Check sheet for the modelled part. Datum: model origin and axes. Units: mm. A direction names the side the tool comes from. Give positions to 0.01 mm unless a question says otherwise; leave off trailing zeros. Order: outer loops, then holes, each group sorted by start corner. A loop starts at its lowest first (then second) coordinate and runs counter-clockwise, first axis right, second up. Notation, with made-up numbers: M -8.75,64.25 L 29.25,64.25 A12 cw 29.25,71.25 Z; hole C 54,79.25 d3. An arc over 180 degrees is marked long. Answer in a Markdown table with one row per item. Add a question column.
from build123d import *

# Parameters (mm, degrees)
ESQUISSE1_W               = 99.5
ESQUISSE1_H               = 12.5
ESQUISSE2_W               = 4.8
ESQUISSE2_H               = 5
ENL_V_MAT_EXTRU_1_DEPTH   = 13.5
SYM_TRIE2_COPY_1_SKETCH_W = 4.8
SYM_TRIE2_COPY_1_SKETCH_H = 5
SYM_TRIE2_COPY_1_DEPTH    = 13.5


with BuildPart() as part:
    # Esquisse1 → Révolution1 (revolve)
    with BuildSketch(Plane.XY, mode=Mode.PRIVATE) as r_volution1_sk:
        with Locations((0, 6.25)):
            Rectangle(ESQUISSE1_W, ESQUISSE1_H)
    revolve(r_volution1_sk.sketch.rotate(Axis((-69.457729469, 0, 0), (1, 0, 0)), 90), axis=Axis((-69.457729469, 0, 0), (1, 0, 0)))  # turned: the seam where the file's is

    # Esquisse2 → Enlèv. mat.-Extru.1 (cut, symmetric)
    with BuildSketch(Plane.XY):
        with Locations((-47.35, 10)):
            Rectangle(ESQUISSE2_W, ESQUISSE2_H)
    enl_v_mat_extru_1 = extrude(amount=ENL_V_MAT_EXTRU_1_DEPTH, both=True, mode=Mode.SUBTRACT)

    # Symétrie1: Enlèv. mat.-Extru.1 across plane
    add(enl_v_mat_extru_1.mirror(Plane.ZX), mode=Mode.SUBTRACT)

    # Esquisse5 → Diamètre du perçage Ø10.5 (10.5)1 (revolve, cut)
    with BuildSketch(Plane(origin=(-49.75, 0, 0), x_dir=(0, 0, 1), z_dir=(0, 1, 0))):
        Polygon((0, 0), (0, 36.15451825), (5.25, 33), (5.25, 0), align=None)
    diam_tre_du_per_age_10_5_10_5_1 = revolve(axis=Axis((-56.1, 0, 0), (1, 0, 0)), mode=Mode.SUBTRACT)

    # Symétrie2: Diamètre du perçage Ø10.5 (10.5)1, Enlèv. mat.-Extru.1 across plane
    add(diam_tre_du_per_age_10_5_10_5_1.mirror(Plane(origin=(0, 0, 0), x_dir=(0, 0, 1), z_dir=(1, 0, 0))), mode=Mode.SUBTRACT)
    add(enl_v_mat_extru_1.mirror(Plane(origin=(0, 0, 0), x_dir=(0, 0, 1), z_dir=(1, 0, 0))), mode=Mode.SUBTRACT)

    # Symétrie2 copy 1 sketch → Symétrie2 copy 1 (cut, symmetric)
    with BuildSketch(Plane(origin=(0, 0, 0), x_dir=(-1, 0, 0), z_dir=(0, 0, 1))):
        with Locations((-47.35, 10)):
            Rectangle(SYM_TRIE2_COPY_1_SKETCH_W, SYM_TRIE2_COPY_1_SKETCH_H)
    extrude(amount=SYM_TRIE2_COPY_1_DEPTH, both=True, mode=Mode.SUBTRACT)


solid = part.part
Q1. Cross-section at B-B (x = -15). Record the boundary of the cut face in (y, z), and give its area (3 significant figures).
Q2. Cross-section at D-D (y = 9.75). Record the boundary of the cut face in (x, z).
Q3. Go/stop test with flat-tipped pins: pin 1 (4 mm diameter, centred on x = -46.5, z = -2.5, fed in from -Y); pin 2 (1.4 mm diameter, centred on x = 46, z = 1.5, fed in from -Y); pin 3 (5 mm diameter, centred on x = 2, y = 5, fed in from -Z). Record where each tip stops, or that it passes through.
Q4. Cross-section at A-A (z = -7). Record the boundary of the cut face in (x, y), and give its area (3 significant figures).
Q5. Draft check along Y on faces 1 (the conical face through (14.143, 0.89, -0.198)), 2 (the flat face through (47, -7.5, 0)), 3 (the flat face through (44.95, -9, 0)). Enter one of: pulls with the +Y half, pulls with the -Y half, needs draft (parallel to the pull), parting line crosses it, or undercut.
Q6. Thickness scan on probe 1 along Y at (x, z) = (35, 0); probe 2 along Z at (x, y) = (-43, -3.5); probe 3 along X at (y, z) = (8, 4.5). Record the ranges inside material, lowest first.
Q7. Cross-section at C-C (x = 9). Record the boundary of the cut face in (y, z).
Q8. Tool access check on faces 4 (the flat face through (-47, -7.5, 0)), 5 (the flat face through (-47, 7.5, 0)), 6 (the flat face through (44.95, 9, 0)), 7 (the cylindrical face through (-33.5, -1.6, 5)), 8 (the cylindrical face through (33.5, -1.6, 5)). Record the directions out of +Z, -Z, +X, -X, +Y, -Y that give a thin tool (end or side, any length) a straight path to the whole face; none if there is none.
Values follow:
| question | item | result |
|---|---|---|
| 1 | outline | C 0,0 d25; hole C 0,0 d4.68 |
| 1 | area | 474 mm² |
| 2 | outline | M -44.95,-7.82 L 44.95,-7.82 L 44.95,7.82 L -44.95,7.82 Z |
| 3 | pin 1 | y = -12.44 |
| 3 | pin 2 | y = -7.5 |
| 3 | pin 3 | z = -12.25 |
| 4 | outline | M -49.75,-7.5 L -44.95,-7.5 L -44.95,-10.36 L 44.95,-10.36 L 44.95,-7.5 L 49.75,-7.5 L 49.75,7.5 L 44.95,7.5 L 44.95,10.36 L -44.95,10.36 L -44.95,7.5 L -49.75,7.5 Z |
| 4 | area | 2,010 mm² |
| 5 | face 1 | undercut |
| 5 | face 2 | pulls with the -Y half |
| 5 | face 3 | needs draft |
| 6 | probe 1 | -12.5 to -5.25, 5.25 to 12.5 |
| 6 | probe 2 | -12 to -3.91, 3.91 to 12 |
| 6 | probe 3 | -44.95 to 44.95 |
| 7 | outline | C 0,0 d25 |
| 8 | face 4 | +Z, -Z, -X, -Y |
| 8 | face 5 | +Z, -Z, -X, +Y |
| 8 | face 6 | +Z, -Z, +X, +Y |
| 8 | face 7 | -X |
| 8 | face 8 | +X |
